CAD build for the part. Positions are in the model's coordinates, mm. Face numbers are marked on the shaded views. A direction names the side the tool comes from. Round coordinates to 2 decimals unless told otherwise and drop trailing zeros. Order: outer loops, then holes, each group sorted by start corner. A loop starts at its lowest first (then second) coordinate and runs counter-clockwise, first axis right, second up. Notation, with made-up numbers: M -6.5,22 L 21.5,22 A13 cw 21.5,47 Z; hole C 8.25,29.5 d4. An arc over 180 degrees is marked long. Answer as a JSON object with one key per item and string values.
```python
from build123d import *

# Parameters (mm, degrees)
F0_W     = 76.2
F0_H     = 101.6
F2_DEPTH = 25.4
F1_R     = 50.8
F3_DEPTH = 25.4
F4_R     = 25.275511
F5_DEPTH = 25.401
F6_W     = 38.1
F6_H     = 101.6
F7_DEPTH = 50.8
F8_W     = 38.1
F8_H     = 73.628832
F9_DEPTH = 76.2


with BuildPart() as f2:
    # F0 (on Top) → F2 (new body)
    with BuildSketch(Plane.XY):
        with Locations((-38.1, 0)):
            Rectangle(F0_W, F0_H)
    extrude(amount=F2_DEPTH)

    # F1 (on Top) → F3 (join)
    with BuildSketch(Plane.XY):
        Circle(F1_R)
    extrude(amount=F3_DEPTH)

    # F4 (on Top) → F5 (cut, through all)
    with BuildSketch(Plane.XY):
        Circle(F4_R)
    extrude(amount=F5_DEPTH, mode=Mode.SUBTRACT)

    # F6 (on Top) → F7 (join)
    with BuildSketch(Plane.XY):
        with Locations((-57.15, 0)):
            Rectangle(F6_W, F6_H)
    extrude(amount=F7_DEPTH)

    # F8 (on Top) → F9 (join)
    with BuildSketch(Plane.XY):
        with Locations((-57.15, 13.985584)):
            Rectangle(F8_W, F8_H)
    extrude(amount=F9_DEPTH)


solid = f2.part
```
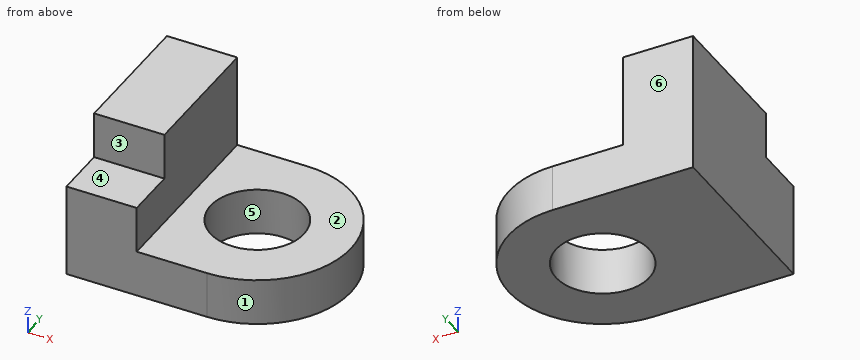
Item 1: Saw through at D-D on z = 30.5. List the corners of the cut face in (x, y), and give its area (3 significant figures).
Worked answers:
{"outline": "M -76.2,-50.8 L -38.1,-50.8 L -38.1,50.8 L -76.2,50.8 Z", "area": "3,870 mm2"}
Item 2: Two-plate mould, pull along Y, no slides. Class the marked faces 4, 5 and 6: released by +Y, released by -Y, zero draft, split by the parting line, or undercut.
Worked answers:
{"face 4": "zero draft", "face 5": "undercut", "face 6": "released by +Y"}
Item 3: Saw through at B-B on z = 12.5. List the corners of the cut face in (x, y), and give its area (3 significant figures).
Worked answers:
{"outline": "M -76.2,-50.8 L 0,-50.8 A50.8 ccw 0,50.8 L -76.2,50.8 Z; hole C 0,0 d50.55", "area": "9,790 mm2"}
Item 4: 3-axis set-ups, long thin cutter, end or side, ignore diameter. For the marked faces 1, 2 and 3: which of +Z, -Z, +X, -X, +Y, -Y reach the whole face in a straight line?
Worked answers:
{"face 1": "+Z, -Z, +X", "face 2": "+Z, +X, +Y, -Y", "face 3": "+Z, +X, -X, -Y"}
Item 5: Saw through at C-C on x = 15. List the corners of the cut face in (y, z), and give its area (3 significant figures).
Worked answers:
{"outline": "M -48.53,0 L -20.34,0 L -20.34,25.4 L -48.53,25.4 Z; M 20.34,0 L 48.53,0 L 48.53,25.4 L 20.34,25.4 Z", "area": "1,430 mm2"}
Item 6: Wall check: line 1 along X through (y, z) = (-1, 5.5); line 2 along Y through (x, z) = (0, 11.25); line 3 along Z through (x, y) = (-4, 43.5). Give the ranges that are in metal, low to high. Write a range as [from, to].
Worked answers:
{"line 1": "x = [-76.2, -25.26], [25.26, 50.79]", "line 2": "y = [-50.8, -25.28], [25.28, 50.8]", "line 3": "z = [0, 25.4]"}
Item 7: Drop flat-ended pins along their axis: pin 1 Ø6 at (x, z) = (21, 23) entering from +Y; pin 2 Ø22.5 at (x, y) = (-53, -39.5) entering from +Z; pin 3 Ø3 at (x, y) = (11.5, 26) entering from +Z; pin 4 Ø10 at (x, z) = (21, 34.5) entering from -Y. Give the stop position or say it passes through.
Worked answers:
{"pin 1": "stops at y = 47.5", "pin 2": "stops at z = 50.8", "pin 3": "stops at z = 25.4", "pin 4": "passes through"}
Item 8: Saw through at A-A on y = 0. List the corners of the cut face in (x, z).
Worked answers:
{"outline": "M -76.2,0 L -25.28,0 L -25.28,25.4 L -38.1,25.4 L -38.1,76.2 L -76.2,76.2 Z; M 25.28,0 L 50.8,0 L 50.8,25.4 L 25.28,25.4 Z"}
